Autodesk Inventor part; units mm, degrees
ref_plane "YZ Plane" through (0, 0, 0) normal (1, 0, 0) x (0, 1, 0)
ref_plane "XZ Plane" through (0, 0, 0) normal (0, 1, 0) x (-1, 0, 0)
ref_plane "XY Plane" through (0, 0, 0) normal (0, 0, 1) x (1, 0, 0)
sketch "Sketch1" plane through (0, 0, 0) normal (0, 1, 0) x (-1, 0, 0)
  line L0 (21, 10.5) -> (-21, 10.5)
  line L1 (-21, 10.5) -> (-21, -10.5)
  line L2 (-21, -10.5) -> (21, -10.5)
  line L3 (21, -10.5) -> (21, 10.5)
  line L4 (21, 10.5) -> (-21, -10.5) construction
  line L5 (-21, 10.5) -> (21, -10.5) construction
  line L6 (-29, 18.5) -> (29, 18.5)
  line L7 (29, 18.5) -> (29, -18.5)
  line L8 (29, -18.5) -> (-29, -18.5)
  line L9 (-29, -18.5) -> (-29, 18.5)
  circle A0 centre (10.5, 14.5) radius 1.75
  line L10 (0, 10.5) -> (0, -10.5) construction
  line L11 (-21, 0) -> (21, 0) construction
  circle A1 centre (10.5, -14.5) radius 1.75
  circle A2 centre (-10.5, 14.5) radius 1.75
  circle A3 centre (-10.5, -14.5) radius 1.75
  line L12 (-21, 10.5) -> (-27, 10.5)
  line L13 (-27, 10.5) -> (-27, -10.5)
  line L14 (-27, -10.5) -> (-21, -10.5)
  line L15 (-21, -10.5) -> (-21, 10.5)
  line L16 (21, 10.5) -> (27, 10.5)
  line L17 (27, 10.5) -> (27, -10.5)
  line L18 (27, -10.5) -> (21, -10.5)
  line L19 (7.75, 10.5) -> (13.25, 10.5)
  line L20 (13.25, 10.5) -> (13.25, 17)
  line L21 (13.25, 17) -> (7.75, 17)
  line L22 (7.75, 17) -> (7.75, 10.5)
  line L23 (-13.25, 10.5) -> (-13.25, 17)
  line L24 (-13.25, 17) -> (-7.75, 17)
  line L25 (-7.75, 17) -> (-7.75, 10.5)
  line L26 (13.25, -10.5) -> (13.25, -17)
  line L27 (13.25, -17) -> (7.75, -17)
  line L28 (7.75, -17) -> (7.75, -10.5)
  line L29 (-7.75, -17) -> (-7.75, -10.5)
  line L30 (-13.25, -17) -> (-7.75, -17)
  line L31 (-13.25, -10.5) -> (-13.25, -17)
  point P0 (0, 0)
  dimension "d0" = 21
  dimension "d1" = 42
  dimension "d2" = 8
  dimension "d3" = 3.5
  dimension "d4" = 10.5
  dimension "d5" = 4
  dimension "d6" = 6
  dimension "d7" = 21
  dimension "d15" = 5.5
  dimension "d17" = 2.5
  dimension "d18" = 2.75
extrude "Extrusion1" add sketch "Sketch1" along normal blind 8 contours L16 L17 L18 L3 | L0 L22 L21 L20 | L26 L27 L28 L2 | L0 L23 L24 L25 | L29 L30 L31 L2 | L1 L14 L13 L12 | L6 L7 L8 L9
fillet "Fillet1" radius 8 2 edges at (-29, 4, 18.5) (29, 4, 18.5)
fillet "Fillet3" radius 2 10 edges at (-26.6569, 0, 16.1569) (0, 0, 18.5) (26.6569, 0, 16.1569) (29, 0, -4) (-29, 0, -4) (-26.6569, 8, 16.1569) (0, 8, 18.5) (26.6569, 8, 16.1569) (29, 8, -4) (-29, 8, -4)
extrude "Extrusion3" cut sketch "Sketch1" along normal blind 2 contours L0 L22 L21 L20 | L26 L27 L28 L2 | L0 L23 L24 L25 | L29 L30 L31 L2
fillet "Fillet4" radius 2 8 edges at (13.25, 1.0318, 17) (7.75, 1.0318, 17) (-13.25, 1.0318, 17) (-7.75, 1.0318, 17) (-13.25, 1, -17) (-7.75, 1, -17) (13.25, 1, -17) (7.75, 1, -17)
fillet "Fillet5" radius 2 8 edges at (-7.75, 1, -10.5) (-13.25, 1, -10.5) (7.75, 1, -10.5) (13.25, 1, -10.5) (13.25, 1, 10.5) (7.75, 1, 10.5) (-7.75, 1, 10.5) (-13.25, 1, 10.5)
equation "\"d0\" = MountWidth"
equation "\"d1\" = MountLength"
equation "\"d2\" = MountThickness"
equation "\"d3\" = THROUGH_DIAMETER"
equation "\"d4\" = 0.25 * MountLength"
equation "\"d5\" = 0.5 * MountThickness"
equation "\"d7\" = MountWidth"
equation "\"d8\" = OUTER_HEIGHT"
equation "\"d12\" = OUTER_FILLET"
equation "\"d14\" = PART_FILLET"
properties part number "CoxaServoCutout"
Could you check a few things on this model? Use its own coordinates, in mm. A direction names the side the tool comes from. Coordinates: 2 decimals unless noted, no trailing zeros. Order: outer loops, then holes, each group sorted by start corner. A loop starts at its lowest first (then second) coordinate and runs counter-clockwise, first axis right, second up. Notation, with made-up numbers: M 33,-20.75 L 68,-20.75 A27 cw 68,-2.75 Z; hole C -12.75,17.25 d8. An arc over 180 degrees is marked long. Use one line per item in the form item = value. Start each with the question number.
1. On a 3-axis mill with a long thin cutter (end or side, diameter ignored), from which of +Z, -Z, +X, -X, +Y, -Y can I reach the whole of each face in a straight line? I mean faces 4 (the cylindrical face through (10.728, 4.958, 12.765)), 5 (the cylindrical face through (12.68, 1.01, -16.4)). Say none if no direction works.
2. For pin 1 (1.6 mm diameter, centred on y = 0.5, z = -14.5, fed in from +X); pin 2 (1.6 mm diameter, centred on y = 1, z = -13.5, fed in from -X); pin 3 (0.6 mm diameter, centred on y = 1, z = 13.5, fed in from -X), each with a flat end and sliding along its axis, tell me the tip position at first contact or that it passes through.
3. Please list where these lines run through material, in increasing order: line 1 (Z direction, x = -10.5, y = 4.5); line 2 (X direction, y = 5, z = 7); line 3 (Z direction, x = -1, y = 4.5).
4. Suppose I cut it at D-D on x = -10.5. Write out the boundary of the cut face in (y, z).
5. Suppose I cut it at A-A on z = -3. Write out the boundary of the cut face in (x, y).
6. Suppose I cut it at B-B on x = -18. Write out the boundary of the cut face in (y, z).
7. Suppose I cut it at C-C on y = 3.25. Write out the boundary of the cut face in (x, z).
8. We'd pull the mould along Z, two halves only. Please class faces 1 (the cylindrical face through (-12.65, 1.01, -16.43)), 2 (the cylindrical face through (-28.4, 0.57, -4.2)), 3 (the cylindrical face through (-0.29, 0.57, 17.9)): +Z half, -Z half, draft (parallel to the pull), parting line (faces both ways), or undercut.
Geometry says:
q1.face_4 = +Y, -Y
q1.face_5 = -Y
q2.pin_1 = 28.87
q2.pin_2 = -28.99
q2.pin_3 = -28.33
q3.line_1 = -18.5 to -16.25, -12.75 to -10.5, 10.5 to 12.75, 16.25 to 18.5
q3.line_2 = -29 to -21, 21 to 29
q3.line_3 = -18.5 to -10.5, 10.5 to 18.5
q4.outline = M 0,-18.5 L 8,-18.5 L 8,-16.25 L 2,-16.25 L 2,-17 L 0,-17 Z; M 0.06,17 L 2,17 L 2,16.25 L 8,16.25 L 8,16.5 A2 ccw 6,18.5 L 2,18.5 A2 ccw Z; M 2,-12.75 L 8,-12.75 L 8,-10.5 L 2,-10.5 Z; M 2,10.5 L 8,10.5 L 8,12.75 L 2,12.75 Z
q5.outline = M -29,2 A2 ccw -27,0 L -21,0 L -21,8 L -27,8 A2 ccw -29,6 Z; M 21,0 L 27,0 A2 ccw 29,2 L 29,6 A2 ccw 27,8 L 21,8 Z
q6.outline = M 0,-18.5 L 8,-18.5 L 8,-10.5 L 0,-10.5 Z; M 0,10.5 L 8,10.5 L 8,16.5 A2 ccw 6,18.5 L 2,18.5 A2 ccw 0,16.5 Z
q7.outline = M -29,-18.5 L 29,-18.5 L 29,10.5 A8 ccw 21,18.5 L -21,18.5 A8 ccw -29,10.5 Z; hole M -21,-10.5 L 21,-10.5 L 21,10.5 L -21,10.5 Z; hole C -10.5,-14.5 d3.5; hole C -10.5,14.5 d3.5; hole C 10.5,-14.5 d3.5; hole C 10.5,14.5 d3.5
q8.face_1 = undercut
q8.face_2 = draft
q8.face_3 = +Z half
